```python
from build123d import *

# Parameters (mm, degrees)
SKETCH3_R                    = 2
CUT_EXTRUDE1_DEPTH           = 28.712812921
M4_CLEARANCE_HOLE1_OUTLINE_W = 2.15
M4_CLEARANCE_HOLE1_OUTLINE_H = 7.500042463
SKETCH13_R                   = 1.5
CUT_EXTRUDE3_DEPTH           = 26.612496997


# Read off the part's stored shape, not the designer's step: M4 Clearance Hole1
with BuildPart() as part:
    # Sketch2 → Revolve1 (revolve)
    with BuildSketch(Plane.XY, mode=Mode.PRIVATE) as revolve1_sk:
        Polygon((0, 22.228628213), (7, 22.228628213), (7.5, 21.728628213), (7.5, 10.228628213), (16, 10.228628213), (16, 6.728628213), (15.5, 6.228628213), (0, 6.228628213), align=None)
    revolve(revolve1_sk.sketch.rotate(Axis((0, 0, 0), (0, 1, 0)), 90), axis=Axis((0, 0, 0), (0, 1, 0)))

    # Sketch3 → Cut-Extrude1 (cut, through all)
    with BuildSketch(Plane(origin=(0, 22.228628213, 0), x_dir=(1, 0, 0), z_dir=(0, 1, 0))):
        with Locations(Location((0, 0, 0), (0, 0, 270))):
            Circle(SKETCH3_R)
    extrude(amount=-CUT_EXTRUDE1_DEPTH, mode=Mode.SUBTRACT)

    # M4 Clearance Hole1 outline → M4 Clearance Hole1 (revolve, cut)
    with BuildSketch(Plane(origin=(0, 16.228628213, 0), x_dir=(0, 1, 0), z_dir=(0, 0, -1))):
        with Locations((1.075, 3.750021232)):
            Rectangle(M4_CLEARANCE_HOLE1_OUTLINE_W, M4_CLEARANCE_HOLE1_OUTLINE_H)
    revolve(axis=Axis((0, 16.228628213, 0), (1, 0, 0)), mode=Mode.SUBTRACT)

    # Sketch13 → Cut-Extrude3 (cut, through all)
    with BuildSketch(Plane(origin=(0, 10.228628213, 0), x_dir=(1, 0, 0), z_dir=(0, 1, 0))):
        with Locations(Location((-12, 0, 0), (0, 0, 270))):
            Circle(SKETCH13_R)
        with Locations(Location((0, 12, 0), (0, 0, 270))):
            Circle(SKETCH13_R)
        with Locations(Location((12, 0, 0), (0, 0, 270))):
            Circle(SKETCH13_R)
        with Locations(Location((0, -12, 0), (0, 0, 270))):
            Circle(SKETCH13_R)
    extrude(amount=-CUT_EXTRUDE3_DEPTH, mode=Mode.SUBTRACT)


solid = part.part
```
Model file for the job. Use its own axes, mm. A direction names the side the tool comes from. Coordinates: 2 decimals unless noted, no trailing zeros. Loops run counter-clockwise (first coordinate to the right, second up) from the corner with the lowest first, then second, coordinate; pieces in that order, holes last. Notation, with made-up numbers: (66, -25) -> (100, -25) arc R13 cw to (100, -10) -> close; hole circle Ø10 at (19, 12.25). An arc over 180 degrees is marked (long way). Answer as a JSON object with one key per item and string values.
Q1. Flat gauge pins, fed straight in: P1, Ø5, axis at y = 8, z = 7, coming from the -X side; P2, Ø5, axis at y = 12, z = 6.5, coming from the +X side; P3, Ø4, axis at x = 4, y = 8.5, coming from the -Z side; P4, Ø1.8, axis at x = 0, z = 12, coming from the -Y side. Where does each tip first touch, or does it go through?
Report:
{"P1": "stops at x = -15.35", "P2": "stops at x = 15.28", "P3": "stops at z = -15.87", "P4": "passes through"}
Q2. Cut at C-C (y = 21). List the corners of the cut face in (x, z).
Report:
{"outline": "circle Ø15 at (0, 0); hole circle Ø4 at (0, 0)"}
Q3. 3-axis set-ups, long thin cutter, end or side, ignore diameter. For faces 4 (the cylindrical face through (4.64, 18.28, 0.65)), 5 (the cylindrical face through (-2, 14, 0)), 6 (the flat face through (3.33, 10.229, 6.89)): which of +Z, -Z, +X, -X, +Y, -Y reach the whole face in a straight line?
Report:
{"face 4": "+X", "face 5": "+Y, -Y", "face 6": "+Y"}
Q4. Cut at A-A (z = 0). List the corners of the cut face in (x, y), and give its area (3 significant figures).
Report:
{"outline": "(-16, 6.73) -> (-15.5, 6.23) -> (-13.5, 6.23) -> (-13.5, 10.23) -> (-16, 10.23) -> close; (-10.5, 6.23) -> (-2, 6.23) -> (-2, 22.23) -> (-7, 22.23) -> (-7.5, 21.73) -> (-7.5, 10.23) -> (-10.5, 10.23) -> close; (2, 6.23) -> (10.5, 6.23) -> (10.5, 10.23) -> (7.5, 10.23) -> (7.5, 14.08) -> (2, 14.08) -> close; (2, 18.38) -> (7.5, 18.38) -> (7.5, 21.73) -> (7, 22.23) -> (2, 22.23) -> close; (13.5, 6.23) -> (15.5, 6.23) -> (16, 6.73) -> (16, 10.23) -> (13.5, 10.23) -> close", "area": "196 mm2"}
Q5. Cut at D-D (y = 16). List the corners of the cut face in (x, z), and give its area (3 significant figures).
Report:
{"outline": "(0, -2.14) -> (0, -2) arc R2 cw to (0, 2) -> (0, 2.14) -> (7.19, 2.14) arc R7.5 ccw (long way) to (7.19, -2.14) -> close", "area": "139 mm2"}
Q6. Probe probe 1 along X at (y, z) = (8.15, 0); probe 2 along Y at (x, z) = (6, 0); probe 3 along Y at (x, z) = (-10, -7). List the from-to ranges inside material, lowest first.
Report:
{"probe 1": "x = -16 to -13.5, -10.5 to -2, 2 to 10.5, 13.5 to 16", "probe 2": "y = 6.23 to 14.08, 18.38 to 22.23", "probe 3": "y = 6.23 to 10.23"}
Q7. Pull direction X, two halves, no side cores. Call faces 1 (the flat face through (3, 6.229, 0)), 2 (the cylindrical face through (-6.324, 15.898, -4.032)), 3 (the cylindrical face through (0.07, 8.26, 10.5)): released by +X, released by -X, zero draft, split by the parting line, or undercut.
Report:
{"face 1": "zero draft", "face 2": "split by the parting line", "face 3": "undercut"}
Q8. Cut at B-B (y = 8.5). List the corners of the cut face in (x, z), and give its area (3 significant figures).
Report:
{"outline": "circle Ø32 at (0, 0); hole circle Ø3 at (-12, 0); hole circle Ø4 at (0, 0); hole circle Ø3 at (0, -12); hole circle Ø3 at (0, 12); hole circle Ø3 at (12, 0)", "area": "763 mm2"}
